Input: part model. Units: mm. Frame: model coordinates. Face numbers are marked on the shaded views. A direction names the side the tool comes from. Give positions to 0.01 mm unless a question says otherwise; leave off trailing zeros. Write each loop counter-clockwise with the first axis right and the second up, starting at its lowest first coordinate (ties: lowest second). Pieces come first, ordered by that corner, then holes. Notation, with made-up numbers: (44.5, -0.75) -> (81.5, -0.75) arc R8 cw to (81.5, 14.25) -> close; hole circle Ø7 at (-33.75, 23). An arc over 180 degrees is marked (long way). Answer as a JSON object with one key per item and string values. Group by question number.
from build123d import *

# Parameters (mm, degrees)
SKETCH_1_W          = 39.9
SKETCH_1_H          = 20
EXTRUDE_1_DEPTH     = 8
SKETCH_2_W          = 39.9
SKETCH_2_H          = 9
CUT_EXTRUDE_1_DEPTH = 4.5
SKETCH_3_R          = 1.5
CUT_EXTRUDE_2_DEPTH = 4


with BuildPart() as part:
    # 草图1 → 凸台-拉伸1 (new body)
    with BuildSketch(Plane(origin=(0, 0, 0), x_dir=(1, 0, 0), z_dir=(0, 1, 0))):
        Rectangle(SKETCH_1_W, SKETCH_1_H)
    extrude(amount=EXTRUDE_1_DEPTH)

    # 草图2 → 切除-拉伸1 (cut)
    with BuildSketch(Plane(origin=(0, 8, 0), x_dir=(1, 0, 0), z_dir=(0, 1, 0))):
        Rectangle(SKETCH_2_W, SKETCH_2_H)
    extrude(amount=-CUT_EXTRUDE_1_DEPTH, mode=Mode.SUBTRACT)

    # 草图3 → 切除-拉伸2 (cut)
    with BuildSketch(Plane.XZ):
        with Locations((-8, 7.5)):
            Circle(SKETCH_3_R)
        with Locations((8, 7.5)):
            Circle(SKETCH_3_R)
        with Locations((8, -7.5)):
            Circle(SKETCH_3_R)
        with Locations((-8, -7.5)):
            Circle(SKETCH_3_R)
    extrude(amount=-CUT_EXTRUDE_2_DEPTH, mode=Mode.SUBTRACT)


solid = part.part
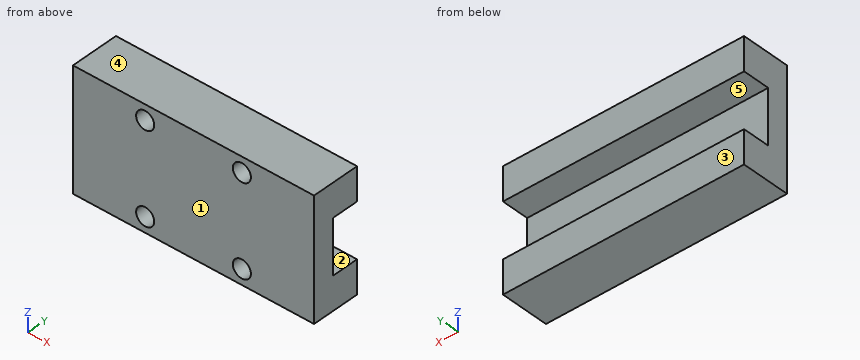
1. Section B-B (y = 5). Return the cut outline in (x, z).
2. Section D-D (z = -7.5). Return the cut outline in (x, y).
3. Reachability of the marked faces 1 and 2 from +Z, -Z, +X, -X, +Y, -Y: full face, straight path, thin tool, end or side. Return the list, or none.
4. Line query: line 1 (Z direction, x = -8, y = 2.25); line 2 (Z direction, x = -17.5, y = 4.75); line 3 (X direction, y = 0.5, z = -6.75). Output: solid intervals per line, ascending.
5. Contact query for flat-ended pins moving along their axis: pin 1 Ø0.9 at (x, z) = (-8, 8) entering from -Y; pin 2 Ø2.5 at (x, z) = (4.5, 1) entering from +Y. Output: stop coordinate, or through.
6. Section C-C (x = -8). Return the cut outline in (y, z), plus the area to 3 significant figures.
7. Mould query, pull axis Z, two halves, no side actions, for the marked faces 3, 4 and 5. Classes: pulls with the +Z half, pulls with the -Z half, needs draft (parallel to the pull), parting line crosses it, or undercut.
8. Section A-A (y = 3). Return the cut outline in (x, z), plus the area to 3 significant figures.
Working result:
{
 "1": {"outline": "(-19.95, -10) -> (19.95, -10) -> (19.95, -4.5) -> (-19.95, -4.5) -> close; (-19.95, 4.5) -> (19.95, 4.5) -> (19.95, 10) -> (-19.95, 10) -> close"},
 "2": {"outline": "(-19.95, 0) -> (-9.5, 0) -> (-9.5, 4) -> (-6.5, 4) -> (-6.5, 0) -> (6.5, 0) -> (6.5, 4) -> (9.5, 4) -> (9.5, 0) -> (19.95, 0) -> (19.95, 8) -> (-19.95, 8) -> close"},
 "3": {"face 1": "+Z, -Z, +X, -X, -Y", "face 2": "+X, -X, +Y"},
 "4": {"line 1": "z = -10 to -9, -6 to 6, 9 to 10", "line 2": "z = -10 to -4.5, 4.5 to 10", "line 3": "x = -19.95 to -9.3, -6.7 to 6.7, 9.3 to 19.95"},
 "5": {"pin 1": "stops at y = 4", "pin 2": "stops at y = 3.5"},
 "6": {"outline": "(0, -10) -> (8, -10) -> (8, -4.5) -> (3.5, -4.5) -> (3.5, 4.5) -> (8, 4.5) -> (8, 10) -> (0, 10) -> (0, 9) -> (4, 9) -> (4, 6) -> (0, 6) -> (0, -6) -> (4, -6) -> (4, -9) -> (0, -9) -> close", "area": "95.5 mm^2"},
 "7": {"face 3": "needs draft", "face 4": "pulls with the +Z half", "face 5": "undercut"},
 "8": {"outline": "(-19.95, -10) -> (19.95, -10) -> (19.95, 10) -> (-19.95, 10) -> close; hole circle Ø3 at (-8, -7.5); hole circle Ø3 at (-8, 7.5); hole circle Ø3 at (8, -7.5); hole circle Ø3 at (8, 7.5)", "area": "770 mm^2"}
}
